Could you check a few things on this model? Use its own coordinates, in mm. Face numbers are marked on the shaded views. A direction names the side the tool comes from. Round coordinates to 2 decimals unless told otherwise and drop trailing zeros. Loops run counter-clockwise (first coordinate to the right, second up) from the corner with the lowest first, then second, coordinate; pieces in that order, holes last. Notation, with made-up numbers: M 60,-10 L 101,-10 A9 ccw 101,-4 Z; hole C -24.5,29.5 d3. An arc over 180 degrees is marked long. One line per item, written item: value. Start each with the question number.
Q1. Imagine slicing it at C-C (x = 17.6). Please give me the cut outline in (y, z), then the cut area to 3 significant figures.
Q2. Which directions (+Z, -Z, +X, -X, +Y, -Y) give clear straight access to the entire face, cutting with the end or side of a thin tool? Please do the marked faces 1, 2 and 3.
Q3. Imagine slicing it at D-D (y = 5). Please give me the cut outline in (x, z).
Q4. I'm going to push flat-ended pins straight in: pin 1 Ø5.5 at (x, y) = (7, 9) entering from +Z; pin 2 Ø0.5 at (x, z) = (17, 5.5) entering from +Y; pin 3 Ø1.5 at (x, y) = (8.5, 9) entering from -Z. Where does each tip first touch, or does it pass through?
Q5. Thinking about a two-plate mould opening in X: for the marked faces 4, 5 and 6, which applies, released by +X, released by -X, zero draft, split by the parting line, or undercut?
Q6. Please list where these lines run through material, in increasing order: line 1 along Y through (x, z) = (36.6, 1.5); line 2 along Z through (x, y) = (35.5, 2.5); line 3 along Y through (x, z) = (22.5, -0.75).
Q7. Imagine slicing it at A-A (y = 15). Please give me the cut outline in (x, z), then the cut area to 3 significant figures.
Autodesk Fusion 360 part; units mm, degrees
sketch "Skizze1" plane through (0, 0, 0) normal (0, 0, 1) x (1, 0, 0)
  line L0 (0, 0) -> (40, 0)
  line L1 (40, 0) -> (40, 18)
  line L2 (40, 18) -> (0, 18)
  line L3 (0, 18) -> (0, 0)
  circle A0 centre (36.6, 15) radius 1.25
  circle A1 centre (17.6, 15) radius 1.25
  line L4 (36.6, 15) -> (17.6, 15) construction
  line L5 (0, 0) -> (40, 0)
  line L6 (40, 0) -> (40, 4)
  line L7 (40, 4) -> (0, 4)
  line L8 (0, 4) -> (0, 0)
  line L9 (0, 18) -> (4, 18)
  line L10 (4, 18) -> (4, 0)
  line L11 (4, 0) -> (0, 0)
  line L12 (0, 0) -> (0, 18)
  line L13 (17.6, 18) -> (17.6, 4) construction
  line L14 (36.6, 18) -> (36.6, 4) construction
  line L15 (15.1, 18) -> (15.1, 4)
  line L16 (34.1, 18) -> (34.1, 4)
  line L17 (20.1, 18) -> (20.1, 4)
  line L18 (4, 17) -> (40, 17)
  dimension "d1" = 40
  dimension "d2" = 18
  dimension "d3" = 19
  dimension "d4" = 2.5
  dimension "d5" = 3
  dimension "d6" = 3.4
  dimension "d7" = 4
  dimension "d8" = 2.5
  dimension "d9" = 5
  dimension "d17" = 1
  dimension "d36" = 4
extrude "Extrusion1" add sketch "Skizze1" along normal blind 4.5
extrude "Extrusion2" cut sketch "Skizze1" against normal blind 2.2 from surface at 4.5 contours L7 L10 L15 L18 | L7 L16 L17 L18
extrude "Extrusion3" add sketch "Skizze1" against normal blind 10 contours L0 L3 L5 L7 L8 L10 L11 L12 | L0 L1 L5 L6 L7 L10
sketch "Skizze2" plane through (0, 0, 0) normal (0, -1, 0) x (1, 0, 0)
  line L0 (40, -10) -> (40, 4.5)
  line L1 (40, 4.5) -> (0, 4.5)
  line L2 (0, 4.5) -> (0, -10)
  line L3 (0, -10) -> (40, -10)
  line L4 (20, -10) -> (20.1, 4.5) construction
  line L5 (40, 0) -> (0, 0) construction
  circle A0 centre (5.0338, -5) radius 1.6
  circle A1 centre (35.0338, -5.2069) radius 1.6
  point P0 (20.1, 4.5)
  dimension "d18" = 3.2
  dimension "d19" = 5
  dimension "d35" = 30
extrude "Extrusion4" cut sketch "Skizze2" against normal through all contours A0 | A1
chamfer "Fase1" distance 2.2 angle 30 2 edges at (9.55, 17, 2.3) (27.1, 17, 2.3) measured on face at (7.7, 17, 3.7667) measured on face at (24.7667, 17, 3.7667)
sketch "Skizze3" plane through (40, 0, 0) normal (1, 0, 0) x (0, 1, 0)
  line L0 (4, 0) -> (18, 0)
  line L1 (18, 0) -> (18, 4.5)
  line L2 (18, 4.5) -> (0, 4.5)
  line L3 (0, 4.5) -> (0, -10)
  line L4 (0, -10) -> (4, -10)
  line L5 (4, -10) -> (4, 0)
  line L6 (0, 4.5) -> (0, 7.6)
  line L7 (0, 7.6) -> (2.8, 7.6)
  line L8 (2.8, 7.6) -> (2.8, 6.1)
  line L9 (2.8, 6.1) -> (1.3, 6.1)
  line L10 (1.3, 6.1) -> (1.3, 4.5)
  point P0 (18, 4.5)
  dimension "d23" = 16.7
  dimension "d24" = 1.6
  dimension "d25" = 1.5
  dimension "d26" = 1.5
extrude "Extrusion5" add sketch "Skizze3" against normal blind 40 contours L2 L6 L7 L8 L9 L10
chamfer "Fase2" distance 1 angle 45 4 edges at (0, 2, -10) (40, 2, -10) (40, 1.4, 7.6) (0, 1.4, 7.6) measured on face at (13.3333, 2.6667, -10) measured on face at (13.3333, 2.6667, -10) measured on face at (26.6667, 0.9333, 7.6) measured on face at (0, 7.7667, 3)
chamfer "Fase2" distance 0.3 angle 45 3 edges at (20, 2.8, 6.1) (40, 18, 2.25) (0, 18, 2.25) measured on face at (26.6667, 2.8, 7.1) measured on face at (40, 7.7667, 3) measured on face at (26.6667, 18, 1.5)
chamfer "Fase2" distance 0.3 angle 45 4 edges at (16.4346, 15.452, 4.5) (35.4346, 15.452, 4.5) (35.4346, 15.452, 0) (16.4346, 15.452, 0) measured on face at (37.0522, 6.3788, 4.5) measured on face at (37.0522, 6.3788, 4.5) measured on face at (37.8484, 14.9377, 3) measured on face at (18.8484, 14.9377, 3)
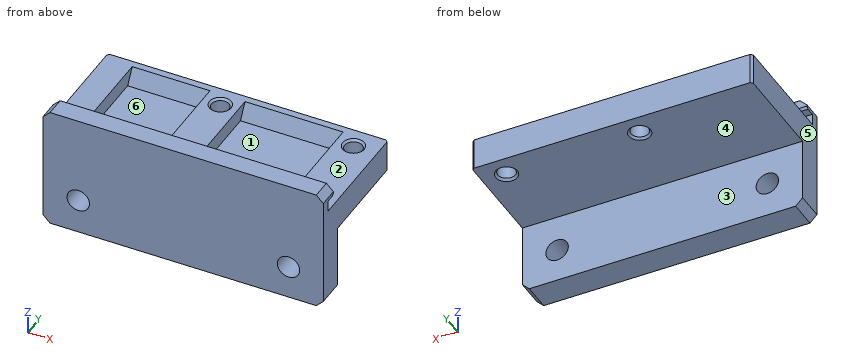
Report:
1. outline: M 0,-10 L 4,-10 L 4,0 L 13.45,0 L 13.75,0.3 L 13.75,4.2 L 13.45,4.5 L 1.3,4.5 L 1.3,6.1 L 2.5,6.1 L 2.8,6.4 L 2.8,7.6 L 0,7.6 Z; M 16.25,0.3 L 16.55,0 L 18,0 L 18,4.5 L 16.55,4.5 L 16.25,4.2 Z
1. area: 116 mm²
2. face 1: +Z
2. face 2: +X, -X, +Y
2. face 3: -Z, +X, -X, +Y
3. outline: M 0,0 L 40,0 L 40,4.5 L 34.1,4.5 L 34.1,2.3 L 20.1,2.3 L 20.1,4.5 L 15.1,4.5 L 15.1,2.3 L 4,2.3 L 4,4.5 L 0,4.5 Z
4. pin 1: stops at z = 2.3
4. pin 2: stops at y = 1.3
4. pin 3: stops at z = 0
5. face 4: zero draft
5. face 5: released by -X
5. face 6: undercut
6. line 1: y = 0 to 13.75, 16.25 to 18
6. line 2: z = -10 to -6.74, -3.68 to 4.5, 6.1 to 7.6
6. line 3: y = 0 to 4
7. outline: M 0,0 L 16.05,0 L 16.35,0.3 L 16.35,4.2 L 16.05,4.5 L 15.1,4.5 L 15.1,2.3 L 4,2.3 L 4,4.5 L 0,4.5 Z; M 18.85,0.3 L 19.15,0 L 35.05,0 L 35.35,0.3 L 35.35,4.2 L 35.05,4.5 L 34.1,4.5 L 34.1,2.3 L 20.1,2.3 L 20.1,4.5 L 19.15,4.5 L 18.85,4.2 Z; M 37.85,0.3 L 38.15,0 L 40,0 L 40,4.5 L 38.15,4.5 L 37.85,4.2 Z
7. area: 102 mm²
